```python
from build123d import *

# Parameters (mm, degrees)
F1_DEPTH = 63.5
F0_W     = 25.3211855178
F0_H     = 19.05
F2_DEPTH = 25.4
F3_DEPTH = 15.875
F5_R     = 6.35


with BuildPart() as f1:
    # F0 (on Front) → F1 (new body, symmetric)
    with BuildSketch(Plane.XZ):
        Polygon((41.275, -9.525), (41.275, 9.525), (22.225, 9.525), (-41.275, 9.525), (-41.275, -9.525), align=None)
    extrude(amount=F1_DEPTH, both=True)

    # F0 (on Front) → F2 (join, symmetric)
    with BuildSketch(Plane.XZ):
        with Locations((72.9855927589, 52.4002)):
            Rectangle(F0_W, F0_H)
        with BuildLine():
            Line((22.225, 9.525), (41.275, 9.525))
            Line((41.275, 9.525), (41.275, 27.0002))
            ThreePointArc((41.275, 27.0002), (45.9246798487, 38.2255201513), (57.15, 42.8752))
            Line((57.15, 42.8752), (60.325, 42.8752))
            Line((60.325, 42.8752), (60.325, 61.9252))
            Line((60.325, 61.9252), (57.15, 61.9252))
            add(Edge.make_bspline(
                [(53.8199176635, 61.7660766125), (54.9516006508, 61.8440010886), (56.0624181193, 61.8973585375), (57.15, 61.9252)],
                knots=[108.144944826, 108.144944826, 108.144944826, 108.144944826, 111.5045361635, 111.5045361635, 111.5045361635, 111.5045361635], degree=3))
            ThreePointArc((53.8199176635, 61.7660766125), (31.3037357574, 50.4890537332), (22.225, 27.0002))
            Line((22.225, 27.0002), (22.225, 9.525))
        make_face()
    extrude(amount=F2_DEPTH, both=True)

    # F0 (on Front) → F3 (join)
    with BuildSketch(Plane.XZ):
        with BuildLine():
            Line((-41.275, 9.525), (22.225, 9.525))
            Line((22.225, 9.525), (22.225, 27.0002))
            ThreePointArc((22.225, 27.0002), (31.3037357574, 50.4890537332), (53.8199176635, 61.7660766125))
            add(Edge.make_bspline(
                [(-41.275, 9.525), (-40.6582798871, 31.2931964034), (17.3911434687, 59.2576946918), (53.8199176635, 61.7660766125)],
                knots=[0, 0, 0, 0, 108.144944826, 108.144944826, 108.144944826, 108.144944826], degree=3))
        make_face()
    extrude(amount=F3_DEPTH)

    # F0 (on Front) → F4 (revolve)
    with BuildSketch(Plane.XZ):
        Polygon((85.725, 52.3875), (85.725, 38.1), (111.125, 38.1), (111.125, 66.675), (85.725, 66.675), align=None)
    revolve(axis=Axis((85.725, 0, 52.3875), (0, 0, -1)))

    # F5
    f5_edges = [f1.edges().sort_by_distance(p)[0] for p in [
        (41.275, 63.5, 0),
        (-41.275, 63.5, 0),
        (41.275, -63.5, 0),
        (-41.275, -63.5, 0),
    ]]
    fillet(f5_edges, radius=F5_R)


solid = f1.part
```
Could you check a few things on this model? Use its own coordinates, in mm. A direction names the side the tool comes from. Round coordinates to 2 decimals unless told otherwise and drop trailing zeros. Loops run counter-clockwise (first coordinate to the right, second up) from the corner with the lowest first, then second, coordinate; pieces in that order, holes last. Notation, with made-up numbers: M -26,1 L -9,1 A18 cw -9,16 Z; hole C -20.75,48.5 d8. An arc over 180 degrees is marked long. Put each result on its own line as item: value.
Q1. Thinking about a two-plate mould opening in X: for faces 4 (the face through (60, 2, 42.875)), 5 (the face through (0, -63.5, 0)), 6 (the face through (-41.275, -1, 0)), which applies, released by +X, released by -X, zero draft, split by the parting line, or undercut?
Check result:
face 4: undercut
face 5: zero draft
face 6: released by -X
Q2. Imagine slicing it at C-C (y = 30.5). Write out the boundary of the cut face in (x, z) (3 decimals), then the cut area to 3 significant figures.
Check result:
outline: M -41.275,-9.525 L 41.275,-9.525 L 41.275,9.525 L -41.275,9.525 Z
area: 1,570 mm2
Q3. Imagine slicing it at B-B (x = 76.5). Write out the boundary of the cut face in (y, z) (3 decimals), then the cut area to 3 significant figures.
Check result:
outline: M -25.4,42.875 L -23.666,42.875 L -23.666,38.1 L 23.666,38.1 L 23.666,42.875 L 25.4,42.875 L 25.4,61.925 L 23.666,61.925 L 23.666,66.675 L -23.666,66.675 L -23.666,61.925 L -25.4,61.925 Z
area: 1,420 mm2
Q4. For pin 1 (14 mm diameter, centred on x = 69, y = 3.5, fed in from -Z); pin 2 (12 mm diameter, centred on y = -31, z = 32.5, fed in from +X); pin 3 (3 mm diameter, centred on x = 51, y = 10.5, fed in from -Z); pin 4 (6 mm diameter, centred on y = 29, z = 50, fed in from +X), each with a flat end and sliding along its axis, tell me the tip position at first contact or that it passes through.
Check result:
pin 1: z = 38.1
pin 2: x = 43.24
pin 3: z = 40.91
pin 4: through
Q5. I need wall thicknesses on probe 1 along Y at (x, z) = (-20.5, 19) (3 decimals); probe 2 along Z at (x, y) = (18.5, -50) (3 decimals); probe 3 along X at (y, z) = (-21, 26) (3 decimals). Which ranges of each line are inside material? Lowest first, please.
Check result:
probe 1: -15.875 to 0
probe 2: -9.525 to 9.525
probe 3: 22.225 to 41.275
Q6. On a 3-axis mill with a long thin cutter (end or side, diameter ignored), from which of +Z, -Z, +X, -X, +Y, -Y can I reach the whole of each face in a straight line? I mean faces 1 (the face through (86, 0, 38.1)), 2 (the face through (60, 0, 61.925)), 3 (the face through (31.548, 12.522, 50.755)). Say none if no direction works.
Check result:
face 1: -Z, +X, +Y, -Y
face 2: +Z, -X
face 3: +Z, -X, +Y
Q7. Imagine slicing it at A-A (z = 6). Write out the boundary of the cut face in (x, y) (3 decimals), then the cut area to 3 significant figures.
Check result:
outline: M -41.275,-57.15 A6.35 ccw -34.925,-63.5 L 34.925,-63.5 A6.35 ccw 41.275,-57.15 L 41.275,57.15 A6.35 ccw 34.925,63.5 L -34.925,63.5 A6.35 ccw -41.275,57.15 Z
area: 10,400 mm2
